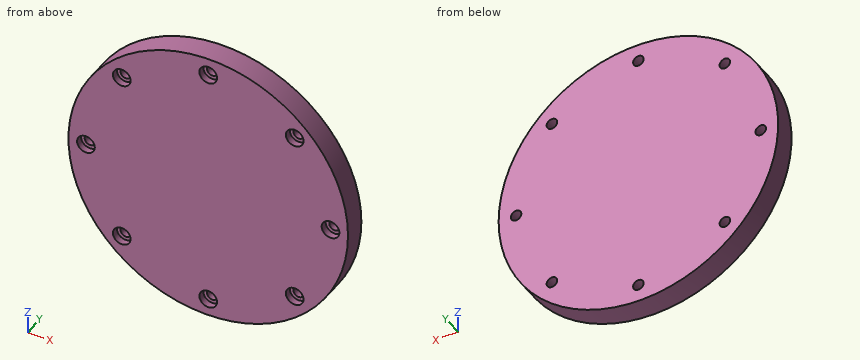
from build123d import *

# Parameters (mm, degrees)
SKETCH1_R                                      = 38.1
BOSS_EXTRUDE1_DEPTH                            = 6.35
CBORE_FOR_4_BUTTON_HEAD_CAP_SCREW1_D           = 2.8702
CBORE_FOR_4_BUTTON_HEAD_CAP_SCREW1_CBORE_D     = 4.826
CBORE_FOR_4_BUTTON_HEAD_CAP_SCREW1_CBORE_DEPTH = 1.905
CIRPATTERN1_COUNT                              = 8


with BuildPart() as part:
    # Sketch1 → Boss-Extrude1 (new body)
    with BuildSketch(Plane(origin=(0, 0, 0), x_dir=(1, 0, 0), z_dir=(0, 1, 0))):
        Circle(SKETCH1_R)
    extrude(amount=BOSS_EXTRUDE1_DEPTH)

    # CBORE for #4 Button Head Cap Screw1 (through all)
    with Locations(Plane(origin=(0, 0, 0), x_dir=(-1, 0, 0), z_dir=(0, -1, 0))):
        with Locations((0, -33.3375)):
            cbore_for_4_button_head_cap_screw1 = CounterBoreHole(CBORE_FOR_4_BUTTON_HEAD_CAP_SCREW1_D / 2, CBORE_FOR_4_BUTTON_HEAD_CAP_SCREW1_CBORE_D / 2, CBORE_FOR_4_BUTTON_HEAD_CAP_SCREW1_CBORE_DEPTH)

    # CirPattern1: CBORE for #4 Button Head Cap Screw1 ×8 about axis
    cirpattern1_axis = Axis((0, 0, 0), (0, 1, 0))
    for i in range(1, CIRPATTERN1_COUNT):
        add(cbore_for_4_button_head_cap_screw1.rotate(cirpattern1_axis, i * 360 / CIRPATTERN1_COUNT), mode=Mode.SUBTRACT)


solid = part.part
Check sheet for the modelled part. Datum: model origin and axes. Units: mm. Give positions to 0.01 mm unless a question says otherwise; leave off trailing zeros. Loops run counter-clockwise (first coordinate to the right, second up) from the corner with the lowest first, then second, coordinate; pieces in that order, holes last. Notation, with made-up numbers: M 84,59 L 99,59 A15 ccw 99,72 Z; hole C -35,53 d2. An arc over 180 degrees is marked long. Answer as a JSON object with one key per item and string values. Group by question number.
Q1. Cross-section at A-A on z = 0. Give the number of separate pieces and of enclosed holes in the cut face, then the cut area to 3 significant figures.
Q2. Cross-section at D-D on z = -14.5. Record the cut outline in (x, y).
Q3. Material ranges on line 1 along X through (y, z) = (4.45, 0); line 2 along X through (y, z) = (1.3, 0), recorded low to high. Write a range as [from, to].
Q4. Go/stop test with flat-tipped pins: P1, Ø2, axis at x = 21.5, y = 4, coming from the -Z side; P2, Ø3.5, axis at x = 0, z = -33.34, coming from the +Y side; P3, Ø3, axis at x = 22, y = 4, coming from the +Z side; P4, Ø1.7, axis at x = 0, z = 33.34, coming from the -Y side. Record where each tip stops, or that it passes through.
Evaluation:
{
 "1": {"separate pieces": "3", "enclosed holes": "0", "area": "440 mm2"},
 "2": {"outline": "M -35.23,0 L 35.23,0 L 35.23,6.35 L -35.23,6.35 Z"},
 "3": {"line 1": "x = [-38.1, -34.77], [-31.9, 31.9], [34.77, 38.1]", "line 2": "x = [-38.1, -35.75], [-30.92, 30.92], [35.75, 38.1]"},
 "4": {"P1": "stops at z = -32.11", "P2": "stops at y = 6.35", "P3": "stops at z = 32.11", "P4": "passes through"}
}
